Autodesk Inventor part; units mm, degrees
ref_plane "YZ Plane" through (0, 0, 0) normal (1, 0, 0) x (0, 1, 0)
ref_plane "XZ Plane" through (0, 0, 0) normal (0, 1, 0) x (-1, 0, 0)
ref_plane "XY Plane" through (0, 0, 0) normal (0, 0, 1) x (1, 0, 0)
sketch "Sketch1" plane through (0, 0, 0) normal (0, 1, 0) x (-1, 0, 0)
  circle A0 centre (0, 0) radius 10.2
  dimension "d0" = 20.4
extrude "Extrusion1" add sketch "Sketch1" along normal blind 25.1
sketch "Sketch2" plane through (0, 25.1, 0) normal (0, 1, 0) x (1, 0, 0)
  circle A0 centre (0, 0) radius 10
  dimension "d3" = 20
extrude "Extrusion2" add sketch "Sketch2" along normal blind 17
sketch "Sketch3" plane through (0, 42.1, 0) normal (0, 1, 0) x (1, 0, 0)
  circle A0 centre (0, 0) radius 3.5
  dimension "d6" = 7
extrude "Extrusion3" add sketch "Sketch3" along normal blind 3
sketch "Sketch4" plane through (0, 45.1, 0) normal (0, 1, 0) x (1, 0, 0)
  circle A0 centre (0, 0) radius 10
  circle A1 centre (0, 0) radius 2
  dimension "d9" = 4
extrude "Extrusion4" add sketch "Sketch4" along normal blind 8 contours A1
sketch "Sketch5" plane through (0, 53.1, 0) normal (0, 1, 0) x (1, 0, 0)
  circle A0 centre (0, 0) radius 2
  circle A1 centre (0, 0) radius 2
  line L0 (-1.5, -1.3229) -> (-1.5, 1.3229)
  point P0 (-2, 0)
  dimension "d12" = 0.5
extrude "Extrusion5" cut sketch "Sketch5" against normal blind 7 contours L0 A0 picked at (-1.5908, -0.3089)
sketch "Sketch6" plane through (0, 42.1, 0) normal (0, 1, 0) x (1, 0, 0)
  circle A0 centre (0, 5.5) radius 1.25
  line L0 (0, 0) -> (3.5, 0) construction
  circle A1 centre (0, 0) radius 3.5
  circle A2 centre (0, -5.5) radius 1.25
  dimension "d15" = 2.5
  dimension "d16" = 11
extrude "Extrusion6" cut sketch "Sketch6" against normal blind 10 contours A0 | A2
properties part number "Stirring motor"
Verification items for the finished model (mm, model axes). A direction names the side the tool comes from. Coordinates: 2 decimals unless noted, no trailing zeros. Order: outer loops, then holes, each group sorted by start corner. A loop starts at its lowest first (then second) coordinate and runs counter-clockwise, first axis right, second up. Notation, with made-up numbers: M 63.25,67.25 L 69.25,67.25 A11 cw 69.25,81.25 Z; hole C 36,2 d3. An arc over 180 degrees is marked long. One line per item, written item: value. Start each with the question number.
Item 1: Depth check by flat-ended pin: P1, Ø0.8, axis at y = 50.5, z = 0, coming from the -X side; P2, Ø2, axis at x = 0, z = -5.5, coming from the +Y side; P3, Ø2, axis at x = -2, z = -3.5, coming from the +Y side. Enter the tip coordinate at first touch or a pass-through.
Item 2: Mould release check, pull along X, two halves, no side actions. Record for faces 1 (the flat face through (0, 53.1, 0)), 2 (the cylindrical face through (-0.27, 37.17, 6.72)), 3 (the cylindrical face through (1.908, 49.044, 0.601)): pulls with the +X half, pulls with the -X half, needs draft (parallel to the pull), parting line crosses it, or undercut.
Item 3: Sectioned sample at B-B on y = 37.5. Record the cut outline in (x, z).
Item 4: Sectioned sample at A-A on z = 0. Record the cut outline in (x, y).
Item 5: Access from +Z, -Z, +X, -X, +Y, -Y to the whole of each face (thin tool, end or side, straight path). Record for faces 4 (the flat face through (0, 32.1, 5)), 5 (the cylindrical face through (-4.707, 12.374, 9.049)), 6 (the flat face through (-1.5, 50, 0)).
Item 6: Thickness scan on probe 1 along Z at (x, y) = (0, 36); probe 2 along Y at (x, z) = (5.5, -2); probe 3 along Y at (x, z) = (1.5, -2.5). Record the ranges inside material, lowest first.
Item 7: Sectioned sample at D-D on y = 22. Record the cut outline in (x, z).
Item 8: Sectioned sample at C-C on x = -3. Record the cut outline in (y, z), then the cut area to 3 significant figures.
Calculated:
1. P1: x = -1.5
1. P2: y = 32.1
1. P3: y = 45.1
2. face 1: needs draft
2. face 2: undercut
2. face 3: parting line crosses it
3. outline: C 0,0 d20; hole C 0,-5.5 d2.5; hole C 0,5.5 d2.5
4. outline: M -10.2,0 L 10.2,0 L 10.2,25.1 L 10,25.1 L 10,42.1 L 3.5,42.1 L 3.5,45.1 L 2,45.1 L 2,53.1 L -1.5,53.1 L -1.5,46.1 L -2,46.1 L -2,45.1 L -3.5,45.1 L -3.5,42.1 L -10,42.1 L -10,25.1 L -10.2,25.1 Z
5. face 4: +Y
5. face 5: +Y, -Y
5. face 6: +Z, -Z, -X, +Y
6. probe 1: -10 to -6.75, -4.25 to 4.25, 6.75 to 10
6. probe 2: 0 to 42.1
6. probe 3: 0 to 45.1
7. outline: C 0,0 d20.4
8. outline: M 0,-9.75 L 25.1,-9.75 L 25.1,-9.54 L 42.1,-9.54 L 42.1,-1.8 L 45.1,-1.8 L 45.1,1.8 L 42.1,1.8 L 42.1,9.54 L 25.1,9.54 L 25.1,9.75 L 0,9.75 Z
8. area: 825 mm^2
